Work out the finished part from the listing and answer in its coordinate system (mm). Coordinates: 2 decimals unless noted, no trailing zeros. Order: outer loops, then holes, each group sorted by start corner. A loop starts at its lowest first (then second) coordinate and runs counter-clockwise, first axis right, second up. Notation, with made-up numbers: M 73,26.5 L 109,26.5 A25 ccw 109,56.5 Z; hole C 40,29 d2. An arc over 180 degrees is marked long. Answer in a Markdown table with one row per item. Add a question column.
Item 1: A flat-ended cylindrical pin translates along its axis: pin 1 Ø1.5 at (x, z) = (7.5, 13) entering from +Y. Find the tip coordinate at first contact, or state that the pin passes through.
Item 2: The part is cut by section A-A (z = 14.5). Write down the section's boundary in (x, y), then the cut area to 3 significant figures.
Item 3: Consider line 1 (X direction, y = 34.5, z = 13.5); line 2 (Y direction, x = 14.5, z = 9.5); line 3 (Y direction, x = 7, z = 5.5). Determine where each line is inside the solid, lowest interval first. Write a range as from..to.
from build123d import *

# Parameters (mm, degrees)
F1_DEPTH = 18.3
F2_R     = 1.5


with BuildPart() as f1:
    # F0 (on Top) → F1 (new body)
    with BuildSketch(Plane.XY):
        with BuildLine():
            ThreePointArc((-11.902175, 2.5), (-11.169942, 0.732233), (-9.402175, 0))
            Line((-9.402175, 0), (15.597825, 0))
            ThreePointArc((15.597825, 0), (17.365592, 0.732233), (18.097825, 2.5))
            Line((18.097825, 2.5), (18.097825, 26.2))
            ThreePointArc((18.097825, 26.2), (3.097825, 41.2), (-11.902175, 26.2))
            Line((-11.902175, 26.2), (-11.902175, 2.5))
        make_face()
    extrude(amount=F1_DEPTH)

    # F2
    f2_edges = [f1.edges().sort_by_distance(p)[0] for p in [
        (-11.902175, 14.35, 18.3),
        (-11.169942, 0.732233, 18.3),
        (3.097825, 0, 18.3),
        (17.365592, 0.732233, 18.3),
        (18.097825, 14.35, 18.3),
        (3.097825, 41.2, 18.3),
    ]]
    fillet(f2_edges, radius=F2_R)


solid = f1.part
Reply:
| question | item | result |
|---|---|---|
| 1 | pin 1 | stops at y = 40.75 |
| 2 | outline | M -11.9,2.5 A2.5 ccw -9.4,0 L 15.6,0 A2.5 ccw 18.1,2.5 L 18.1,26.2 A15 ccw -11.9,26.2 Z |
| 2 | area | 1,140 mm2 |
| 3 | line 1 | x = -9.4..15.59 |
| 3 | line 2 | y = 0..35.95 |
| 3 | line 3 | y = 0..40.68 |
